The drawing under review shows one solid part. Ordinate dimensions are in mm from its lowest x, y, z. Coordinates: 2 decimals unless noted, no trailing zeros. Loops run counter-clockwise (first coordinate to the right, second up) from the corner with the lowest first, then second, coordinate; pieces in that order, holes last. Notation, with made-up numbers: (24, -12.75) -> (81, -12.75) arc R16 ccw to (81, 0.25) -> close; hole circle Ø9 at (87, 51.25). An arc over 180 degrees is marked (long way). Use a Markdown table: item, result.
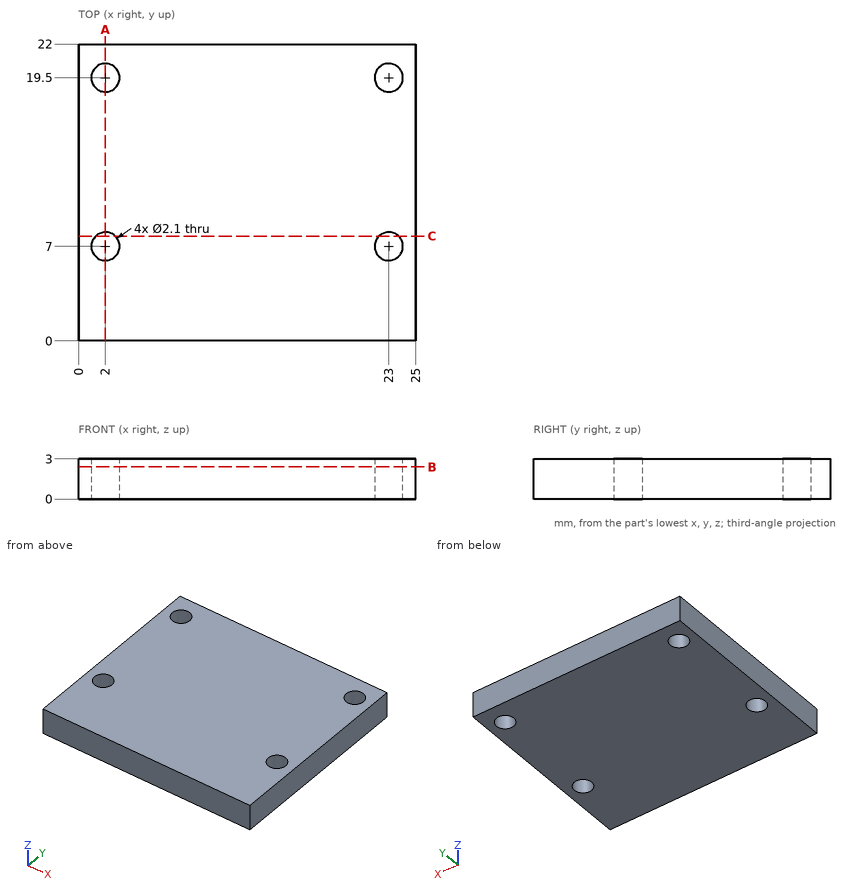
(1) Take a section at B-B on z = 2.4. Write out the cut boundary in (x, y), plus the area to 3 significant figures.
Found:
| item | result |
|---|---|
| outline | (0, 0) -> (25, 0) -> (25, 22) -> (0, 22) -> close; hole circle Ø2.1 at (2, 7); hole circle Ø2.1 at (2, 19.5); hole circle Ø2.1 at (23, 7); hole circle Ø2.1 at (23, 19.5) |
| area | 536 mm^2 |
(2) Take a section at A-A on x = 2. Write out the cut boundary in (y, z), plus the area to 3 significant figures.
Found:
| item | result |
|---|---|
| outline | (0, 0) -> (5.95, 0) -> (5.95, 3) -> (0, 3) -> close; (8.05, 0) -> (18.45, 0) -> (18.45, 3) -> (8.05, 3) -> close; (20.55, 0) -> (22, 0) -> (22, 3) -> (20.55, 3) -> close |
| area | 53.4 mm^2 |
(3) Take a section at C-C on y = 7.75. Write out the cut boundary in (x, z), plus the area to 3 significant figures.
Found:
| item | result |
|---|---|
| outline | (0, 0) -> (1.27, 0) -> (1.27, 3) -> (0, 3) -> close; (2.73, 0) -> (22.27, 0) -> (22.27, 3) -> (2.73, 3) -> close; (23.73, 0) -> (25, 0) -> (25, 3) -> (23.73, 3) -> close |
| area | 66.2 mm^2 |
(4) For pin 1 Ø2.5 at (x, y) = (23, 7) entering from -Z, flat-tipped, find the tip position at first contact; note if it passes through.
Found:
| item | result |
|---|---|
| pin 1 | stops at z = 0 |
(5) For line 1 along Y through (x, z) = (2, 0.9), list the stretches that pass through material, from the lowest coordinate up.
Found:
| item | result |
|---|---|
| line 1 | y = 0 to 5.95, 8.05 to 18.45, 20.55 to 22 |
